from build123d import *

# Parameters (mm, degrees)
SKETCH001_W     = 197
SKETCH001_H     = 173
PAD_DEPTH       = 110
SKETCH_W        = 177
SKETCH_H        = 153
POCKET_DEPTH    = 100
SKETCH002_W     = 23.5
SKETCH002_H     = 12
POCKET001_DEPTH = 20
SKETCH003_W     = 35
SKETCH003_H     = 35
POCKET002_DEPTH = 8


with BuildPart() as part:
    # Sketch001 → Pad (new body)
    with BuildSketch(Plane.XY):
        Rectangle(SKETCH001_W, SKETCH001_H)
    extrude(amount=PAD_DEPTH)

    # Sketch (on Face6 of Pad) → Pocket (cut)
    with BuildSketch(Plane.XY.offset(110)):
        Rectangle(SKETCH_W, SKETCH_H)
    extrude(amount=-POCKET_DEPTH, mode=Mode.SUBTRACT)

    # Sketch002 (on Face2 of Pocket) → Pocket001 (cut)
    with BuildSketch(Plane(origin=(-98.5, 0, 0), x_dir=(0, -1, 0), z_dir=(-1, 0, 0))):
        with Locations((0, 54.75)):
            Rectangle(SKETCH002_W, SKETCH002_H)
    extrude(amount=-POCKET001_DEPTH, mode=Mode.SUBTRACT)

    # Sketch003 (on Face11 of Pocket001) → Pocket002 (cut)
    with BuildSketch(Plane.YZ.offset(-88.5)):
        with Locations((0, 55)):
            Rectangle(SKETCH003_W, SKETCH003_H)
    extrude(amount=-POCKET002_DEPTH, mode=Mode.SUBTRACT)


solid = part.part
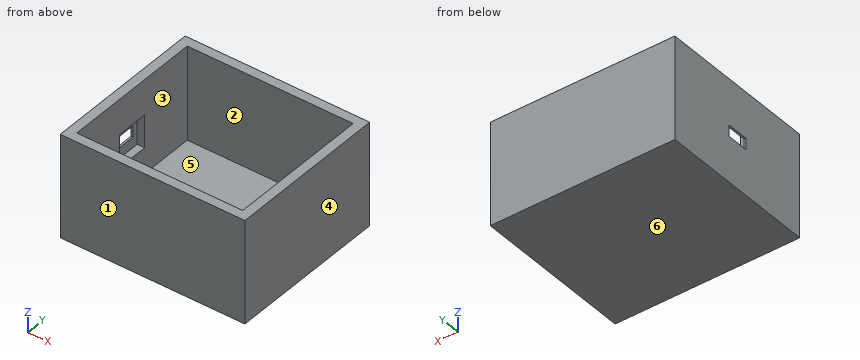
Design review of the part built by this model. Coordinates are the model's own, in mm. Face numbers are marked on the shaded views. A direction names the side the tool comes from. Coordinates: 2 decimals unless noted, no trailing zeros. Loops run counter-clockwise (first coordinate to the right, second up) from the corner with the lowest first, then second, coordinate; pieces in that order, holes last. Notation, with made-up numbers: (18.25, 73.5) -> (57.25, 73.5) arc R15 ccw to (57.25, 83.5) -> close; hole circle Ø8 at (-33, 23). An arc over 180 degrees is marked (long way). Use a Markdown table: item, result. Add a question column.
Item 1: Wall thickness on L1, parallel to X at y = -56, z = 18; L2, parallel to Y at x = -82, z = 102; L3, parallel to X at y = -5.5, z = 69.5: over which ranges is each line inside the solid? List them lowest first. Write a range as from..to.
Item 2: We need section A-A, the plane z = 96. Write out the cut boundary in (x, y).
Item 3: Machinability: for the marked faces 5 and 6, which of the approach directions +Z, -Z, +X, -X, +Y, -Y give a long, thin tool a straight path to every point of the face, cutting with its end or side? Answer none if there is none.
Item 4: We need section C-C, the plane x = 80. Write out the cut boundary in (y, z), and give its area (3 significant figures).
Item 5: Clearance check with a flat-ended pin moving along its axis: P1, Ø1, axis at x = 2.5, y = 37, coming from the +Z side. State where the tip first meets the part, or that it passes through.
Item 6: The part is to be moulded in two halves that separate along Y. For the marked faces 1, 2, 3 and 4, say which applies: +Y half, -Y half, draft (parallel to the pull), parting line (faces both ways), or undercut.
Item 7: We need section B-B, the plane y = -34.5. Write out the cut boundary in (x, z).
Numbers:
| question | item | result |
|---|---|---|
| 1 | L1 | x = -98.5..-88.5, 88.5..98.5 |
| 1 | L2 | y = -86.5..-76.5, 76.5..86.5 |
| 1 | L3 | x = -98.5..-96.5, 88.5..98.5 |
| 2 | outline | (-98.5, -86.5) -> (98.5, -86.5) -> (98.5, 86.5) -> (-98.5, 86.5) -> close; hole (-88.5, -76.5) -> (88.5, -76.5) -> (88.5, 76.5) -> (-88.5, 76.5) -> close |
| 3 | face 5 | +Z |
| 3 | face 6 | -Z, +X, -X, +Y, -Y |
| 4 | outline | (-86.5, 0) -> (86.5, 0) -> (86.5, 110) -> (76.5, 110) -> (76.5, 10) -> (-76.5, 10) -> (-76.5, 110) -> (-86.5, 110) -> close |
| 4 | area | 3,730 mm^2 |
| 5 | P1 | stops at z = 10 |
| 6 | face 1 | -Y half |
| 6 | face 2 | undercut |
| 6 | face 3 | undercut |
| 6 | face 4 | draft |
| 7 | outline | (-98.5, 0) -> (98.5, 0) -> (98.5, 110) -> (88.5, 110) -> (88.5, 10) -> (-88.5, 10) -> (-88.5, 110) -> (-98.5, 110) -> close |
